Input: part model. Units: mm. Frame: model coordinates. A direction names the side the tool comes from. Give positions to 0.01 mm unless a question says otherwise; leave off trailing zeros. Order: outer loops, then holes, each group sorted by start corner. A loop starts at its lowest first (then second) coordinate and runs counter-clockwise, first axis right, second up. Notation, with made-up numbers: (30, -2.75) -> (42, -2.75) arc R14 ccw to (42, 6.25) -> close; hole circle Ø7 at (-35, 52). An arc over 180 degrees is marked (long way). Use a Markdown table: item, result. Add a question column.
Autodesk Inventor part; units mm, degrees
ref_plane "YZ Plane" through (0, 0, 0) normal (1, 0, 0) x (0, 1, 0)
ref_plane "XZ Plane" through (0, 0, 0) normal (0, 1, 0) x (-1, 0, 0)
ref_plane "XY Plane" through (0, 0, 0) normal (0, 0, 1) x (1, 0, 0)
sketch "Эскиз1" plane through (0, 0, 0) normal (0, 1, 0) x (-1, 0, 0)
  line L0 (-23, 13.2791) -> (0, 26.5581)
  line L1 (0, 26.5581) -> (23, 13.2791)
  line L2 (23, 13.2791) -> (23, -13.2791)
  line L3 (23, -13.2791) -> (0, -26.5581)
  line L4 (0, -26.5581) -> (-23, -13.2791)
  line L5 (-23, -13.2791) -> (-23, 13.2791)
  line L6 (0, 0) -> (15.979, 0)
  line L7 (0, 0) -> (15.979, 0) construction
  line L8 (31, -17.8979) -> (31, 17.8979)
  line L9 (31, 17.8979) -> (0, 35.7957)
  line L10 (0, 35.7957) -> (-31, 17.8979)
  line L11 (-31, 17.8979) -> (-31, -17.8979)
  line L12 (-31, -17.8979) -> (0, -35.7957)
  line L13 (0, -35.7957) -> (31, -17.8979)
  dimension "d2" = 46
  dimension "d3" = 8
extrude "Выдавливание1" add sketch "Эскиз1" along normal blind 7.5
sketch "Эскиз2" plane through (0, 7.5, 0) normal (0, 1, 0) x (1, 0, 0)
  line L0 (31, -17.8979) -> (31, 17.8979)
  line L1 (31, 17.8979) -> (31, -17.8979)
  line L2 (31, -17.8979) -> (0, -35.7957)
  line L3 (0, -35.7957) -> (-31, -17.8979)
  line L4 (-31, -17.8979) -> (-31, 17.8979)
  line L5 (-31, 17.8979) -> (0, 35.7957)
  line L6 (0, 35.7957) -> (31, 17.8979)
  circle A0 centre (0, 0) radius 12.5
  point P0 (31, -17.8979)
  dimension "d6" = 25
extrude "Выдавливание2" add sketch "Эскиз2" along normal blind 2
sketch "Эскиз3" plane through (0, 0, 0) normal (0, -1, 0) x (1, 0, 0)
  line L0 (0, 35.7957) -> (31, 17.8979) construction
  line L1 (15.5, 26.8468) -> (11.5, 19.9186) construction
  line L2 (23, 13.2791) -> (0, 26.5581) construction
  circle A0 centre (13.5, 23.3827) radius 2
  circle A1 centre (0, 0) radius 27 construction
  circle A2 centre (-13.5, 23.3827) radius 2
  circle A3 centre (-27, 0) radius 2
  circle A4 centre (-13.5, -23.3827) radius 2
  circle A5 centre (13.5, -23.3827) radius 2
  circle A6 centre (27, 0) radius 2
  dimension "d9" = 4
  dimension "d12" = 360
extrude "Выдавливание3" cut sketch "Эскиз3" against normal blind 4
properties part number "держатель"
Q1. Access query for faces 5 (the flat face through (11.661, 3.698, 19.826)), 6 (the flat face through (-31, 5, 0)). Directions: +Z, -Z, +X, -X, +Y, -Y. A direction counts if a zero-diameter tool reaches every point of the face in a straight line with its end or side. Return the directions, or none.
Q2. Section query B-B (z = -19.5). Return loops of the section in (x, y), plus the area to 3 significant figures.
Q3. Section query A-A (x = -6). Return loops of the section in (y, z), plus the area to 3 significant figures.
Q4. Ray query, line 1 (X direction, y = 2, z = -13); line 2 (Z direction, x = 0, y = 1.5); line 3 (Z direction, x = 13.5, y = 0.85). Return the intervals inside material, ascending.
Q5. Draft query along Z for faces 1 (the flat face through (15.283, 4.684, 26.972)), 2 (the flat face through (-15.283, 4.684, -26.972)), 3 (the flat face through (31, 5, 0)), 4 (the flat face through (27, 4, 0)). Return one class per face: +Z half, -Z half, draft (parallel to the pull), parting line (faces both ways), or undercut.
Q6. Section query D-D (z = 14.5). Return loops of the section in (x, y).
Q7. Section query C-C (x = 13.5). Return loops of the section in (y, z), plus the area to 3 significant figures.
Q8. First-contact query: pin 1 (2.5 mm diameter, centred on x = 27, z = 0, fed in from -Y); pin 2 (10 mm diameter, centred on x = -12.5, z = -10.5, fed in from -Y); pin 3 (3 mm diameter, centred on x = 14, y = 3.5, fed in from -Z). Flat tips, straight axial feed; report the tip coordinate or a pass-through.
Solution:
| question | item | result |
|---|---|---|
| 1 | face 5 | -Y |
| 1 | face 6 | +Z, -Z, -X, +Y, -Y |
| 2 | outline | (-28.23, 0) -> (-12.23, 0) -> (-12.23, 7.5) -> (12.23, 7.5) -> (12.23, 0) -> (28.23, 0) -> (28.23, 9.5) -> (-28.23, 9.5) -> close |
| 2 | area | 353 mm² |
| 3 | outline | (0, -32.33) -> (9.5, -32.33) -> (9.5, -10.97) -> (7.5, -10.97) -> (7.5, -23.09) -> (0, -23.09) -> close; (0, 23.09) -> (7.5, 23.09) -> (7.5, 10.97) -> (9.5, 10.97) -> (9.5, 32.33) -> (0, 32.33) -> close |
| 3 | area | 224 mm² |
| 4 | line 1 | x = -31 to -23, 23 to 31 |
| 4 | line 2 | z = -35.8 to -26.56, 26.56 to 35.8 |
| 4 | line 3 | z = -28 to -25.38, -21.38 to -18.76, 18.76 to 21.38, 25.38 to 28 |
| 5 | face 1 | +Z half |
| 5 | face 2 | -Z half |
| 5 | face 3 | draft |
| 5 | face 4 | undercut |
| 6 | outline | (-31, 0) -> (-20.89, 0) -> (-20.89, 7.5) -> (20.89, 7.5) -> (20.89, 0) -> (31, 0) -> (31, 9.5) -> (-31, 9.5) -> close |
| 7 | outline | (0, -28) -> (9.5, -28) -> (9.5, 28) -> (0, 28) -> (0, 25.38) -> (4, 25.38) -> (4, 21.38) -> (0, 21.38) -> (0, 18.76) -> (7.5, 18.76) -> (7.5, -18.76) -> (0, -18.76) -> (0, -21.38) -> (4, -21.38) -> (4, -25.38) -> (0, -25.38) -> close |
| 7 | area | 219 mm² |
| 8 | pin 1 | stops at y = 4 |
| 8 | pin 2 | stops at y = 7.5 |
| 8 | pin 3 | stops at z = -28.58 |
